Here's how the part is built. I have some questions about the finished solid (model axes, mm). A direction names the side the tool comes from. Round coordinates to 2 decimals unless told otherwise and drop trailing zeros. Loops run counter-clockwise (first coordinate to the right, second up) from the corner with the lowest first, then second, coordinate; pieces in that order, holes last. Notation, with made-up numbers: (5.25, 51) -> (21.25, 51) arc R9 cw to (21.25, 56) -> close; hole circle Ø4 at (84.25, 12). An arc over 180 degrees is marked (long way). Use one line per item in the form item = value. Start each with the question number.
Item 1: I'm going to push flat-ended pins straight in: pin 1 Ø5 at (x, z) = (30.5, 200.5) entering from -Y; pin 2 Ø6 at (x, y) = (-46.5, -70.5) entering from -Z; pin 3 Ø6 at (x, y) = (62, -68) entering from +Z; pin 4 Ø1.6 at (x, z) = (83.5, 146.5) entering from -Y. Where does each tip first touch, or does it pass through?
Item 2: If I drill on L1, parallel to X at y = -32, z = 309; L2, parallel to X at y = 38.1, z = 309.3; L3, parallel to Z at x = -41, y = 38.6, over which ranges is the centre line in solid material (lowest first)? Write a range as [from, to].
Item 3: If we section it at A-A (y = 26.5): Write out the boundary of the cut face in (x, z), then the cut area to 3 significant figures.
Item 4: If we section it at B-B (x = 0): Write out the boundary of the cut face in (y, z), then the cut area to 3 significant figures.
Item 5: Thinking about a two-plate mould opening in X: for faces 4 (the face through (1, -25, 520)), 5 (the face through (60.794, -66.185, 518.986)), 6 (the face through (1, -26, 518)), 7 (the face through (-60.21, -66.77, 518.99)), which applies, released by +X, released by -X, zero draft, split by the parting line, or undercut?
Item 6: If we section it at C-C (z = 364.3): Write out the boundary of the cut face in (x, y), then the cut area to 3 significant figures.
Item 7: If we section it at D-D (z = 35): Write out the boundary of the cut face in (x, y), then the cut area to 3 significant figures.
Item 8: For faces 1 (the face through (82.5, -4, 256)), 2 (the face through (-1, 37.521, 255)), 3 (the face through (-83.51, -23.48, 461.77)), which set-ups out of +Z, -Z, +X, -X, +Y, -Y let a thin tool reach every point of the face, with its end or its side?
```python
from build123d import *

# Parameters (mm, degrees)
FLANGE_BASE1_DEPTH                 = 520
ESBO_O6_R                          = 5
CORTE_EXTRUS_O4_DEPTH              = 10
ARESTA_FLANGE1_STRIP_W             = 10
ARESTA_FLANGE1_STRIP_H             = 2
ARESTA_FLANGE1_STRIP_CUT_DEPTH     = 163
ARESTA_FLANGE1_DEPTH               = 163
QUEBRA_CANTO1_START                = 518
QUEBRA_CANTO1_DEPTH                = 2
ESBO_O10_R                         = 17.5
CORTE_EXTRUS_O5_DEPTH              = 10
FILETE1_R                          = 10
ESBO_O11_R                         = 5
CORTE_EXTRUS_O6_DEPTH              = 4
FURO_DE_DI_METRO_10_5_10_5_1_D     = 10.5
FURO_DE_DI_METRO_10_5_10_5_1_DEPTH = 11
FURO_DE_DI_METRO_10_5_10_5_1_TIP   = 3.15451825


# Read off the part's stored shape, not the designer's step: Quebra-Canto1
# Sheet-metal steps are written as plain solids
with BuildPart() as part:
    # Esboço1 → Flange-base1 (new body)
    with BuildSketch(Plane.XY):
        with BuildLine():
            Line((-82.5, -44.978989098), (-82.5, 36.521010902))
            ThreePointArc((-82.5, 36.521010902), (-82.207106781, 37.228117683), (-81.5, 37.521010902))
            Line((-81.5, 37.521010902), (81.5, 37.521010902))
            ThreePointArc((81.5, 37.521010902), (82.207106781, 37.228117683), (82.5, 36.521010902))
            Line((82.5, 36.521010902), (82.5, -44.978989098))
            Line((82.5, -44.978989098), (84.5, -44.978989098))
            Line((84.5, -44.978989098), (84.5, 36.521010902))
            ThreePointArc((84.5, 36.521010902), (83.621320344, 38.642331245), (81.5, 39.521010902))
            Line((81.5, 39.521010902), (-81.5, 39.521010902))
            ThreePointArc((-81.5, 39.521010902), (-83.621320344, 38.642331245), (-84.5, 36.521010902))
            Line((-84.5, 36.521010902), (-84.5, -44.978989098))
            Line((-84.5, -44.978989098), (-82.5, -44.978989098))
        make_face()
    extrude(amount=FLANGE_BASE1_DEPTH)

    # Esboço6 → Corte-extrusão4 (cut)
    with BuildSketch(Plane(origin=(0, 39.521010902, 0), x_dir=(1, 0, 0), z_dir=(0, 1, 0))):
        with Locations(Location((47, -485, 0), (0, 0, 180))):
            Circle(ESBO_O6_R)
        with Locations(Location((47, -35, 0), (0, 0, 180))):
            Circle(ESBO_O6_R)
        with Locations((-47, -485)):
            Circle(ESBO_O6_R)
        with Locations((-47, -35)):
            Circle(ESBO_O6_R)
    extrude(amount=-CORTE_EXTRUS_O4_DEPTH, mode=Mode.SUBTRACT)

    # Aresta-Flange1 strip (across the edge) → Aresta-Flange1 strip cut (cut)
    with BuildSketch(Plane(origin=(81.5, 37.521010902, 520), x_dir=(0, 0, -1), z_dir=(-1, 0, 0))):
        with Locations((-2, -1)):
            Rectangle(ARESTA_FLANGE1_STRIP_W, ARESTA_FLANGE1_STRIP_H)
    extrude(amount=ARESTA_FLANGE1_STRIP_CUT_DEPTH, mode=Mode.SUBTRACT)

    # Aresta-Flange1 section (across the edge) → Aresta-Flange1 (add)
    with BuildSketch(Plane(origin=(81.5, 37.521010902, 520), x_dir=(0, 0, -1), z_dir=(-1, 0, 0))):
        with BuildLine():
            Line((0, 1), (0, 125))
            Line((0, 125), (2, 125))
            Line((2, 125), (2, 1))
            ThreePointArc((2, 1), (2.292893219, 0.292893219), (3, 0))
            Line((3, 0), (3, -2))
            ThreePointArc((3, -2), (0.878679656, -1.121320344), (0, 1))
        make_face()
    extrude(amount=ARESTA_FLANGE1_DEPTH)

    # Quebra-Canto1 outline → Quebra-Canto1 (cut)
    with BuildSketch(Plane.XY.offset(QUEBRA_CANTO1_START)):
        Polygon((81.5, -87.478989098), (81.5, -45.478989098), (39.5, -87.478989098), align=None)
        Polygon((-81.5, -87.478989098), (-39.5, -87.478989098), (-81.5, -45.478989098), align=None)
    extrude(amount=QUEBRA_CANTO1_DEPTH, mode=Mode.SUBTRACT)

    # Esboço10 → Corte-extrusão5 (cut)
    with BuildSketch(Plane.XY.offset(520)):
        with Locations((0, -47.478989098)):
            Circle(ESBO_O10_R)
    extrude(amount=-CORTE_EXTRUS_O5_DEPTH, mode=Mode.SUBTRACT)

    # Filete1
    filete1_edges = [part.edges().sort_by_distance(p)[0] for p in [
        (83.5, -44.978989098, 0),
        (-83.5, -44.978989098, 0),
    ]]
    fillet(filete1_edges, radius=FILETE1_R)

    # Esboço11 → Corte-extrusão6 (cut)
    with BuildSketch(Plane.ZY.offset(84.5)):
        with Locations((457, -24.978989098)):
            Circle(ESBO_O11_R)
    extrude(amount=-CORTE_EXTRUS_O6_DEPTH, mode=Mode.SUBTRACT)

    # Furo de diâmetro Ø10.5 (10.5)1
    with Locations(Plane(origin=(-41, 39.521010902, 364.3), x_dir=(1, 0, 0), z_dir=(0, 1, 0))):
        with Locations((0, 0), (82, 0), (82, 55), (0, 55)):
            Hole(FURO_DE_DI_METRO_10_5_10_5_1_D / 2, depth=FURO_DE_DI_METRO_10_5_10_5_1_DEPTH)
            with Locations((0, 0, -(FURO_DE_DI_METRO_10_5_10_5_1_DEPTH + FURO_DE_DI_METRO_10_5_10_5_1_TIP / 2))):  # 118° drill point
                Cone(0, FURO_DE_DI_METRO_10_5_10_5_1_D / 2, FURO_DE_DI_METRO_10_5_10_5_1_TIP, mode=Mode.SUBTRACT)


solid = part.part
```
Values found:
q1.pin_1 = 37.52
q1.pin_2 = 518
q1.pin_3 = 520
q1.pin_4 = -44.98
q2.L1 = [-84.5, -82.5], [82.5, 84.5]
q2.L2 = [-84.05, -46.25], [-35.75, 35.75], [46.25, 84.05]
q2.L3 = [0, 304.05], [314.55, 359.05], [369.55, 519.16]
q3.outline = (-84.5, 0) -> (-82.5, 0) -> (-82.5, 520) -> (-84.5, 520) -> close; (-81.5, 518) -> (81.5, 518) -> (81.5, 520) -> (-81.5, 520) -> close; (82.5, 0) -> (84.5, 0) -> (84.5, 520) -> (82.5, 520) -> close
q3.area = 2,410 mm2
q4.outline = (-87.48, 518) -> (-64.98, 518) -> (-64.98, 520) -> (-87.48, 520) -> close; (-29.98, 518) -> (36.52, 518) arc R1 cw to (37.52, 517) -> (37.52, 0) -> (39.52, 0) -> (39.52, 517) arc R3 ccw to (36.52, 520) -> (-29.98, 520) -> close
q4.area = 1,220 mm2
q5.face_4 = zero draft
q5.face_5 = released by +X
q5.face_6 = undercut
q5.face_7 = released by -X
q6.outline = (-84.5, -44.98) -> (-82.5, -44.98) -> (-82.5, 36.52) arc R1 cw to (-81.5, 37.52) -> (-46.25, 37.52) -> (-46.25, 39.52) -> (-81.5, 39.52) arc R3 ccw to (-84.5, 36.52) -> close; (-35.75, 37.52) -> (35.75, 37.52) -> (35.75, 39.52) -> (-35.75, 39.52) -> close; (46.25, 37.52) -> (81.5, 37.52) arc R1 cw to (82.5, 36.52) -> (82.5, -44.98) -> (84.5, -44.98) -> (84.5, 36.52) arc R3 ccw to (81.5, 39.52) -> (46.25, 39.52) -> close
q6.area = 623 mm2
q7.outline = (-84.5, -44.98) -> (-82.5, -44.98) -> (-82.5, 36.52) arc R1 cw to (-81.5, 37.52) -> (-52, 37.52) -> (-52, 39.52) -> (-81.5, 39.52) arc R3 ccw to (-84.5, 36.52) -> close; (-42, 37.52) -> (42, 37.52) -> (42, 39.52) -> (-42, 39.52) -> close; (52, 37.52) -> (81.5, 37.52) arc R1 cw to (82.5, 36.52) -> (82.5, -44.98) -> (84.5, -44.98) -> (84.5, 36.52) arc R3 ccw to (81.5, 39.52) -> (52, 39.52) -> close
q7.area = 625 mm2
q8.face_1 = +Z, -Z, -Y
q8.face_2 = -Z, -Y
q8.face_3 = -X
